Solid Edge part; units mm, degrees
sketch "Sketch1" plane through (0, 0, 0) normal (0, -1, 0) x (1, 0, 0)
  line L0 (-30, 0) -> (-5, 0)
  line L1 (-5, 0) -> (-5, -130)
  line L2 (-5, -130) -> (-15, -130)
  line L3 (-15, -130) -> (-15, -10)
  line L4 (-15, -10) -> (-30, -10)
  line L5 (-30, -10) -> (-30, 0)
  dimension "D1" = 30
  dimension "D2" = 15
revolve "RevolvedProtrusion1" add sketch "Sketch1" angle 360 about axis through (0, 0, 54) along (0, 0, -1)
sketch "Sketch2" plane through (0, 0, -130) normal (0, 0, -1) x (0, 1, 0)
  circle A0 centre (0, 0) radius 10
  circle A1 centre (0, 0) radius 15
extrude "Cutout1" cut sketch "Sketch2" against normal blind 20
cosmetic_thread "Thread1"
sketch "Sketch3" plane through (0, 0, 0) normal (0, 0, 1) x (1, 0, 0)
  circle A0 centre (0, 0) radius 30
  circle A1 centre (0, 0) radius 5
extrude "Ausprägung_1" add sketch "Sketch3" along normal blind 30
sketch "Sketch4" plane through (0, 0, 0) normal (0, 0, 1) x (1, 0, 0)
  line L0 (-61, 50) -> (-11, 50)
  line L1 (-11, 50) -> (-11, -50)
  line L2 (-11, -50) -> (-61, -50)
  line L3 (-61, -50) -> (-61, 50)
extrude "Cutout2" cut sketch "Sketch4" along normal up to next
mirror "Mirror1" about plane through (0, 0, 0) normal (1, 0, 0) of "Cutout2"
hole "Bohrung_1" at (11, -20, 15) direction (-1, 0, 0) diameter 10 end through all
hole "Hole1" at (11, 20, 15) direction (-1, 0, 0) diameter 10 end through all
extrude "Cutout4" [suppressed]
chamfer "Fase_2" distance 1 angle 45 2 edges at (0, -15, -110) (0, -10, -130)
chamfer "Fase_3" distance 1 angle 45 2 edges at (-5, 0, 30) (5, 0, -130)
properties material "Stahl"
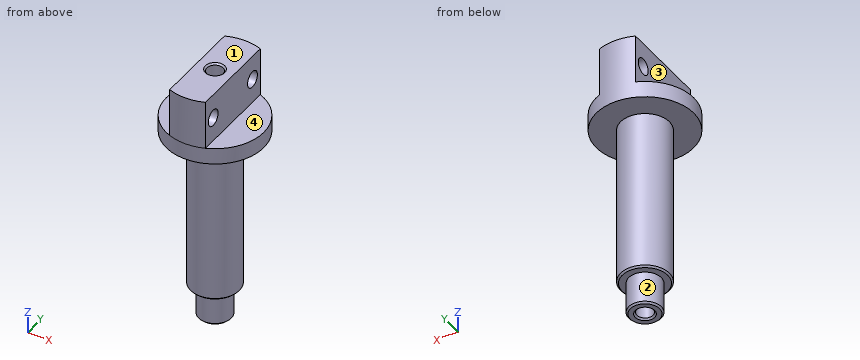
The model under review builds one solid part; all positions refer to its coordinate system, in mm. Face numbers are marked on the shaded views. A direction names the side the tool comes from. Round coordinates to 2 decimals unless told otherwise and drop trailing zeros. Loops run counter-clockwise (first coordinate to the right, second up) from the corner with the lowest first, then second, coordinate; pieces in that order, holes last.
1) Tool access review of the marked faces 1, 2, 3 and 4: name each direction out of +Z, -Z, +X, -X, +Y, -Y from which nothing blocks a thin tool from reaching the whole face with its end or side.
Values follow:
face 1: +Z, +X, -X, +Y, -Y
face 2: -Z
face 3: +Z, -X, +Y, -Y
face 4: +Z, +X, +Y, -Y
2) Consider section B-B on z = -28.5. State the section outline as (x, y) points, then the cut area to 3 significant figures.
Values follow:
outline: circle Ø30 at (0, 0); hole circle Ø10 at (0, 0)
area: 628 mm2
3) Wall thickness on line 1 along Z through (x, y) = (-4, 20); line 2 along X through (y, z) = (0, -77); line 3 along X through (y, z) = (0, 18): over which ranges is each line inside the solid? List them lowest first.
Values follow:
line 1: z = -10 to 10, 20 to 30
line 2: x = -15 to -5, 5 to 15
line 3: x = -11 to -5, 5 to 11
4) Consider section C-C on y = 20. State the section outline as (x, z) points.
Values follow:
outline: (-22.36, -10) - (22.36, -10) - (22.36, 0) - (11, 0) - (11, 10) - (-11, 10) - (-11, 0) - (-22.36, 0) - close; (-11, 20) - (11, 20) - (11, 30) - (-11, 30) - close
5) Consider section D-D on x = -20. State the section outline as (y, z) points.
Values follow:
outline: (-22.36, -10) - (22.36, -10) - (22.36, 0) - (-22.36, 0) - close
6) Clearance check with flat-ended pins moving along their axes: P1, Ø24, axis at y = 2.5, z = 19.5, coming from the -X side; P2, Ø6, axis at x = 3.5, z = 6.5, coming from the -Y side; P3, Ø12, axis at x = -17, y = 0, coming from the -Z side; P4, Ø3, axis at y = -17.5, z = -37.5, coming from the -X side. State where each tip first meets the part, or that it passes through.
Values follow:
P1: stops at x = -11
P2: stops at y = -30
P3: stops at z = -110
P4: passes through
7) Consider section A-A on y = 0. State the section outline as (x, z) points, then the cut area to 3 significant figures.
Values follow:
outline: (-30, -10) - (-15, -10) - (-15, -109) - (-14, -110) - (-10, -110) - (-10, -129) - (-9, -130) - (-6, -130) - (-5, -129) - (-5, 29) - (-6, 30) - (-11, 30) - (-11, 0) - (-30, 0) - close; (5, -129) - (6, -130) - (9, -130) - (10, -129) - (10, -110) - (14, -110) - (15, -109) - (15, -10) - (30, -10) - (30, 0) - (11, 0) - (11, 30) - (6, 30) - (5, 29) - close
area: 3,060 mm2
